Part model, mm, in its own coordinate system. Give positions to 0.01 mm unless a question says otherwise; leave off trailing zeros. Write each loop counter-clockwise with the first axis right and the second up, starting at its lowest first coordinate (ties: lowest second). Pieces come first, ordered by that corner, then holes.
from build123d import *

# Parameters (mm, degrees)
SKETCH1_R           = 2.5
BOSS_EXTRUDE1_DEPTH = 2.5


with BuildPart() as part:
    # Sketch1 → Boss-Extrude1 (new body)
    with BuildSketch(Plane(origin=(0, 0, -1.25), x_dir=(-1, 0, 0), z_dir=(0, 0, -1))):
        Polygon((-3.402954744, -12.7), (50.546, -12.7), (56.896, -6.35), (56.896, 6.35), (50.546, 12.7), (-14.274477372, 50.12412006), (-22.948738686, 52.448381374), (-33.947261314, 46.098381374), (-36.271522628, 37.42412006), (-9.297045256, -9.297045256), align=None)
        with Locations((12.7, 0)):
            Circle(SKETCH1_R, mode=Mode.SUBTRACT)
        with Locations((25.4, 0)):
            Circle(SKETCH1_R, mode=Mode.SUBTRACT)
        Circle(SKETCH1_R, mode=Mode.SUBTRACT)
        with Locations((50.8, 0)):
            Circle(SKETCH1_R, mode=Mode.SUBTRACT)
        with Locations((38.1, 0)):
            Circle(SKETCH1_R, mode=Mode.SUBTRACT)
        with Locations((-25.4, 43.994090512)):
            Circle(SKETCH1_R, mode=Mode.SUBTRACT)
        with Locations((-19.05, 32.995567884)):
            Circle(SKETCH1_R, mode=Mode.SUBTRACT)
        with Locations((-12.7, 21.997045256)):
            Circle(SKETCH1_R, mode=Mode.SUBTRACT)
        with Locations((-6.35, 10.998522628)):
            Circle(SKETCH1_R, mode=Mode.SUBTRACT)
    extrude(amount=-BOSS_EXTRUDE1_DEPTH)


solid = part.part
1) Saw through at B-B (y = 0). Write the cut outline in (x, z), and give its area (3 significant figures).
Check result:
outline: (-56.9, -1.25) - (-53.3, -1.25) - (-53.3, 1.25) - (-56.9, 1.25) - close; (-48.3, -1.25) - (-40.6, -1.25) - (-40.6, 1.25) - (-48.3, 1.25) - close; (-35.6, -1.25) - (-27.9, -1.25) - (-27.9, 1.25) - (-35.6, 1.25) - close; (-22.9, -1.25) - (-15.2, -1.25) - (-15.2, 1.25) - (-22.9, 1.25) - close; (-10.2, -1.25) - (-2.5, -1.25) - (-2.5, 1.25) - (-10.2, 1.25) - close; (2.5, -1.25) - (14.66, -1.25) - (14.66, 1.25) - (2.5, 1.25) - close
area: 116 mm2
2) Saw through at D-D (x = -25). Write the cut outline in (y, z), and give its area (3 significant figures).
Check result:
outline: (-12.7, -1.25) - (-2.47, -1.25) - (-2.47, 1.25) - (-12.7, 1.25) - close; (2.47, -1.25) - (27.45, -1.25) - (27.45, 1.25) - (2.47, 1.25) - close
area: 88.0 mm2
3) Mould opens along X. For faces 1 (the cylindrical face through (17.7, 35.1, 0)), 2 (the cylindrical face through (13.025, 24.476, -0.018)), 3 (the flat face through (-18.59, 31.15, -0.02)), 4 (the flat face through (35.1, 41.8, 0)) say: +X half, -X half, draft (parallel to the pull), parting line (faces both ways), or undercut.
Check result:
face 1: undercut
face 2: undercut
face 3: -X half
face 4: +X half
4) Saw through at A-A (x = 12.7). Write the cut outline in (y, z).
Check result:
outline: (-3.4, -1.25) - (19.5, -1.25) - (19.5, 1.25) - (-3.4, 1.25) - close; (24.5, -1.25) - (49.22, -1.25) - (49.22, 1.25) - (24.5, 1.25) - close
5) Saw through at C-C (z = -0.75). State how many separate pieces and enclosed holes the cut face has, and give its area (3 significant figures).
Check result:
separate pieces: 1
enclosed holes: 9
area: 3,430 mm2
6) Drill centre lines: L1, parallel to X at y = 1.5, z = 0.7; L2, parallel to Y at x = 0, z = -0.35; L3, parallel to X at y = -1, z = 0.45. Where is each one in solid material? Low to high.
Check result:
L1: x = -56.9 to -52.8, -48.8 to -40.1, -36.1 to -27.4, -23.4 to -14.7, -10.7 to -2, 2 to 15.53
L2: y = -12.7 to -2.5, 2.5 to 41.88
L3: x = -56.9 to -53.09, -48.51 to -40.39, -35.81 to -27.69, -23.11 to -14.99, -10.41 to -2.29, 2.29 to 14.09
7) Flat gauge pin, fed straight in: P1, Ø1, axis at x = -2.5, y = 42, coming from the +Z side. Where does the tip first touch, or does it go through?
Check result:
P1: passes through
